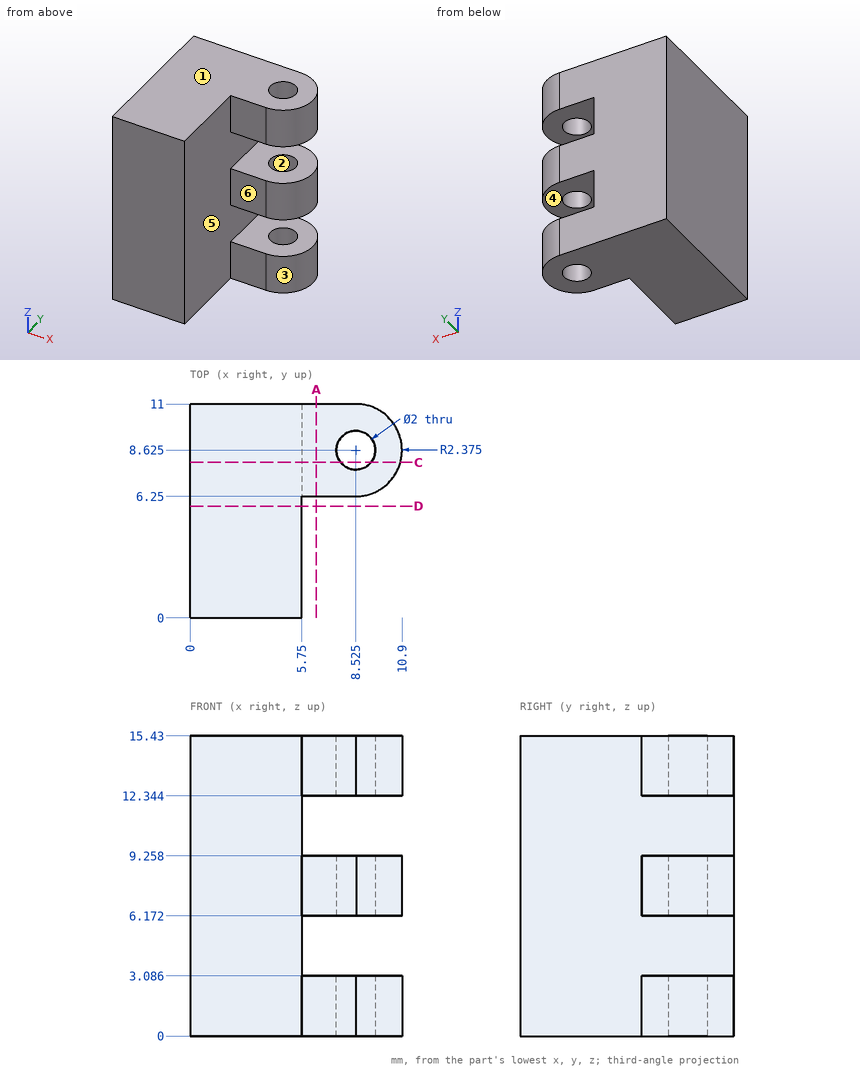
Check sheet for the drawn part. Datum: minimum x, y, z corner. Units: mm. A direction names the side the tool comes from. Round coordinates to 2 decimals unless told otherwise and drop trailing zeros. Loops run counter-clockwise (first coordinate to the right, second up) from the corner with the lowest first, then second, coordinate; pieces in that order, holes last.
Item 1: Gauge pin test, flat ends, axial feed: pin 1 (4 mm diameter, centred on x = 8.5, y = 3.5, fed in from +Z); pin 2 (1 mm diameter, centred on y = 8.5, z = 10.5, fed in from +X); pin 3 (0.8 mm diameter, centred on x = 7, z = 1, fed in from -Y). Record the tip position at first contact, or that the pin passes through.
Item 2: Cross-section at C-C on y = 8. Record the boundary of the cut face in (x, z), then the cut area to 3 significant figures.
Item 3: Cross-section at D-D on y = 5.75. Record the boundary of the cut face in (x, z), then the cut area to 3 significant figures.
Item 4: Thickness scan on line 1 (Z direction, x = 6.5, y = 8.75); line 2 (X direction, y = 1, z = 7); line 3 (X direction, y = 9.5, z = 6.25). Record the ranges inside material, lowest first.
Item 5: Mould release check, pull along X, two halves, no side actions. Record for the marked faces 1, 2 and 3: pulls with the +X half, pulls with the -X half, needs draft (parallel to the pull), parting line crosses it, or undercut.
Item 6: Access from +Z, -Z, +X, -X, +Y, -Y to the whole of each face (thin tool, end or side, straight path). Record for the marked faces 4, 5 and 6.
Item 7: Cross-section at A-A on x = 6.5. Record the boundary of the cut face in (y, z).
Answer sheet:
1. pin 1: passes through
1. pin 2: stops at x = 5.75
1. pin 3: stops at y = 6.25
2. outline: (0, 0) - (7.74, 0) - (7.74, 3.09) - (5.75, 3.09) - (5.75, 6.17) - (7.74, 6.17) - (7.74, 9.26) - (5.75, 9.26) - (5.75, 12.34) - (7.74, 12.34) - (7.74, 15.43) - (0, 15.43) - close; (9.31, 0) - (10.82, 0) - (10.82, 3.09) - (9.31, 3.09) - close; (9.31, 6.17) - (10.82, 6.17) - (10.82, 9.26) - (9.31, 9.26) - close; (9.31, 12.34) - (10.82, 12.34) - (10.82, 15.43) - (9.31, 15.43) - close
2. area: 121 mm2
3. outline: (0, 0) - (5.75, 0) - (5.75, 15.43) - (0, 15.43) - close
3. area: 88.7 mm2
4. line 1: z = 0 to 3.09, 6.17 to 9.26, 12.34 to 15.43
4. line 2: x = 0 to 5.75
4. line 3: x = 0 to 8.04, 9.01 to 10.73
5. face 1: needs draft
5. face 2: undercut
5. face 3: pulls with the +X half
6. face 4: +X, +Y, -Y
6. face 5: +X, -Y
6. face 6: +Z, -Z, +X, -Y
7. outline: (6.25, 0) - (11, 0) - (11, 3.09) - (6.25, 3.09) - close; (6.25, 6.17) - (11, 6.17) - (11, 9.26) - (6.25, 9.26) - close; (6.25, 12.34) - (11, 12.34) - (11, 15.43) - (6.25, 15.43) - close
